```python
from build123d import *
from build123d.topology import SkipClean

# Parameters (mm, degrees)
BASE_FLANGE1_DEPTH     = 3.175
SKETCHED_START         = -76.863629597
SKETCHED_BEND1_DEPTH   = 317.5
SKETCHED_BEND1_2_DEPTH = 101.6
SKETCHED_START_2       = 139.036370403
SKETCHED_BEND1_3_DEPTH = 101.6
SKETCHED_START_3       = 24.736370403
SKETCHED_BEND1_4_DEPTH = 114.3
SKETCHED_BEND1_5_DEPTH = 317.5


# Read off the part's stored shape, not the designer's step: Sketched Bend1
# Sheet-metal steps are written as plain solids
with BuildPart() as part:
    # Sketch1 → Base-Flange1 (new body)
    with BuildSketch(Plane.XY):
        Polygon((-43.155335008, 139.036370403), (-144.755335008, 139.036370403), (-144.755335008, 240.636370403), (-378.435335008, 240.636370403), (-378.435335008, 139.036370403), (-480.035335008, 139.036370403), (-480.035335008, 24.736370403), (-378.435335008, 24.736370403), (-378.435335008, -76.863629597), (-144.755335008, -76.863629597), (-144.755335008, 24.736370403), (-43.155335008, 24.736370403), align=None)
    extrude(amount=-BASE_FLANGE1_DEPTH)

    # Sketched Bend1 outline → Sketched Bend1 (cut)
    with BuildSketch(Plane(origin=(0, 0, 0), x_dir=(1, 0, 0), z_dir=(0, 1, 0)).offset(SKETCHED_START)):
        with BuildLine():
            ThreePointArc((-380.313137759, 0), (-378.20567356, 2.316816086), (-375.193604089, 3.175))
            Line((-375.193604089, 3.175), (-480.035335008, 3.175))
            Line((-480.035335008, 3.175), (-480.035335008, 0))
            Line((-480.035335008, 0), (-380.313137759, 0))
        make_face()
        with BuildLine():
            ThreePointArc((-147.997065928, 3.175), (-144.984996457, 2.316816087), (-142.877532258, 0))
            Line((-142.877532258, 0), (-43.155335008, 0))
            Line((-43.155335008, 0), (-43.155335008, 3.175))
            Line((-43.155335008, 3.175), (-147.997065928, 3.175))
        make_face()
    extrude(amount=SKETCHED_BEND1_DEPTH, mode=Mode.SUBTRACT)

    # Sketched Bend1 2 outline → Sketched Bend1 2 (cut)
    with BuildSketch(Plane(origin=(0, 0, 0), x_dir=(1, 0, 0), z_dir=(0, 1, 0)).offset(SKETCHED_START)):
        Polygon((-377.733604089, 0), (-378.435335008, 0.701730919), (-378.435335008, 0), align=None)
        Polygon((-144.755335008, 0.701730919), (-145.457065927, 0), (-144.755335008, 0), align=None)
    extrude(amount=SKETCHED_BEND1_2_DEPTH, mode=Mode.SUBTRACT)

    # Sketched Bend1 3 outline → Sketched Bend1 3 (cut)
    with BuildSketch(Plane(origin=(0, 0, 0), x_dir=(1, 0, 0), z_dir=(0, 1, 0)).offset(SKETCHED_START_2)):
        Polygon((-377.733604089, 0), (-378.435335008, 0.701730919), (-378.435335008, 0), align=None)
        Polygon((-144.755335008, 0.701730919), (-145.457065927, 0), (-144.755335008, 0), align=None)
    extrude(amount=SKETCHED_BEND1_3_DEPTH, mode=Mode.SUBTRACT)

    # Sketched Bend1 4 outline → Sketched Bend1 4 (add)
    with BuildSketch(Plane(origin=(0, 0, 0), x_dir=(1, 0, 0), z_dir=(0, 1, 0)).offset(SKETCHED_START_3)):
        with BuildLine():
            ThreePointArc((-380.313137759, 0), (-380.757746427, -1.235567159), (-380.908604089, -2.54))
            Line((-380.908604089, -2.54), (-380.908604089, -100.898269081))
            Line((-380.908604089, -100.898269081), (-377.733604089, -100.898269081))
            Line((-377.733604089, -100.898269081), (-377.733604089, -2.54))
            ThreePointArc((-377.733604089, -2.54), (-376.989655313, -0.743948776), (-375.193604089, 0))
            Line((-375.193604089, 0), (-380.313137759, 0))
        make_face()
        with BuildLine():
            ThreePointArc((-147.997065928, 0), (-146.201014704, -0.743948775), (-145.457065928, -2.54))
            Line((-145.457065928, -2.54), (-145.457065928, -100.898269081))
            Line((-145.457065928, -100.898269081), (-142.282065928, -100.898269081))
            Line((-142.282065928, -100.898269081), (-142.282065928, -2.54))
            ThreePointArc((-142.282065928, -2.54), (-142.43292359, -1.235567159), (-142.877532258, 0))
            Line((-142.877532258, 0), (-147.997065928, 0))
        make_face()
    extrude(amount=SKETCHED_BEND1_4_DEPTH)

    # Sketched Bend1 5 outline → Sketched Bend1 5 (add)
    with SkipClean():  # the faces are left unmerged after this step: merging them gives an invalid solid
        with BuildSketch(Plane(origin=(0, 0, 0), x_dir=(1, 0, 0), z_dir=(0, 1, 0)).offset(SKETCHED_START)):
            with BuildLine():
                ThreePointArc((-378.435335008, 2.166634216), (-378.850199632, 1.852099045), (-379.234719343, 1.501115254))
                Line((-379.234719343, 1.501115254), (-378.435335008, 0.701730919))
                Line((-378.435335008, 0.701730919), (-378.435335008, 2.166634216))
            make_face()
            with BuildLine():
                Line((-375.193604089, 0), (-377.733604089, 0))
                Line((-377.733604089, 0), (-376.989655313, -0.743948776))
                ThreePointArc((-376.989655313, -0.743948776), (-376.165620007, -0.193345988), (-375.193604089, 0))
            make_face()
            with BuildLine():
                Line((-145.457065927, 0), (-147.997065928, 0))
                ThreePointArc((-147.997065928, 0), (-147.025050009, -0.193345987), (-146.201014703, -0.743948776))
                Line((-146.201014703, -0.743948776), (-145.457065927, 0))
            make_face()
            with BuildLine():
                ThreePointArc((-143.955950673, 1.501115254), (-144.340470384, 1.852099046), (-144.755335008, 2.166634216))
                Line((-144.755335008, 2.166634216), (-144.755335008, 0.701730919))
                Line((-144.755335008, 0.701730919), (-143.955950673, 1.501115254))
            make_face()
        extrude(amount=SKETCHED_BEND1_5_DEPTH)


solid = part.part
```
Verification items for the finished model (mm, model axes). A direction names the side the tool comes from. Coordinates: 2 decimals unless noted, no trailing zeros. Write each loop counter-clockwise with the first axis right and the second up, starting at its lowest first coordinate (ties: lowest second). Pieces come first, ordered by that corner, then holes. Notation, with made-up numbers: M -18.75,-34 L -6.75,-34 A20 ccw -6.75,2 Z; hole C -30,60.25 d11. An arc over 180 degrees is marked long. Answer as a JSON object with one key per item and string values. Group by question number.
(1) Cross-section at A-A, the plane z = 26. Record the cut outline in (x, y), and give its area (3 significant figures).
(2) Cross-section at C-C, the plane x = -166. Record the cut outline in (y, z) (3 decimals), and give its area (3 significant figures).
(3) Release check for a two-part mould opening along X. For faces 1 (the face through (-377.734, 81, 52)), 2 (the face through (-145.457, 81, 51)), 3 (the face through (-142.282, 81, 52)), 4 (the face through (-380.909, 81, 51)) record: +X half, -X half, draft (parallel to the pull), parting line (faces both ways), or undercut.
(4) Material ranges on line 1 (X direction, y = 36, z = 73); line 2 (Z direction, x = -311, y = -60.5) (3 decimals), recorded low to high.
(5) Cross-section at B-B, the plane y = 160. Record the cut outline in (x, z) (3 decimals), and give its area (3 significant figures).
(6) Tool access check on faces 5 (the face through (-263, 84, 0)), 6 (the face through (-263, 84, -3.175)). Record the directions out of +Z, -Z, +X, -X, +Y, -Y that give a thin tool (end or side, any length) a straight path to the whole face; none if there is none.
(7) Cross-section at D-D, the plane y = 53.5. Record the cut outline in (x, z) (3 decimals).
(8) Gauge pin test, flat ends, axial feed: pin 1 (3 mm diameter, centred on x = -145, z = 50, fed in from +Y); pin 2 (1.2 mm diameter, centred on x = -379, z = 24, fed in from -Y). Record the tip position at first contact, or that the pin passes through.
Reply:
{
 "1": {"outline": "M -380.91,24.74 L -377.73,24.74 L -377.73,139.04 L -380.91,139.04 Z; M -145.46,24.74 L -142.28,24.74 L -142.28,139.04 L -145.46,139.04 Z", "area": "726 mm²"},
 "2": {"outline": "M -76.864,-3.175 L 240.636,-3.175 L 240.636,0 L -76.864,0 Z", "area": "1,010 mm²"},
 "3": {"face 1": "undercut", "face 2": "undercut", "face 3": "+X half", "face 4": "-X half"},
 "4": {"line 1": "-380.91 to -377.73, -145.46 to -142.28", "line 2": "-3.175 to 0"},
 "5": {"outline": "M -379.235,-1.501 A5.715 ccw -375.194,-3.175 L -147.997,-3.175 A5.715 ccw -143.956,-1.501 L -146.201,0.744 A2.54 cw -147.997,0 L -375.194,0 A2.54 cw -376.99,0.744 Z", "area": "742 mm²"},
 "6": {"face 5": "+Z, +Y, -Y", "face 6": "-Z, +X, -X, +Y, -Y"},
 "7": {"outline": "M -380.909,2.54 A5.715 ccw -375.194,-3.175 L -147.997,-3.175 A5.715 ccw -142.282,2.54 L -142.282,100.898 L -145.457,100.898 L -145.457,2.54 A2.54 cw -147.997,0 L -375.194,0 A2.54 cw -377.734,2.54 L -377.734,100.898 L -380.909,100.898 Z"},
 "8": {"pin 1": "y = 139.04", "pin 2": "y = 24.74"}
}
